Build history of the part. All positions in model axes, mm. Face numbers are marked on the shaded views. Coordinates: 2 decimals unless noted, no trailing zeros. Order: outer loops, then holes, each group sorted by start corner. A loop starts at its lowest first (then second) coordinate and runs counter-clockwise, first axis right, second up. Notation, with made-up numbers: (45.5, -31) -> (73.5, -31) arc R29 cw to (73.5, -8) -> close; hole circle Ø10 at (66, 49). An arc over 180 degrees is marked (long way). Write each question's results on one line, items separated by ' | '.
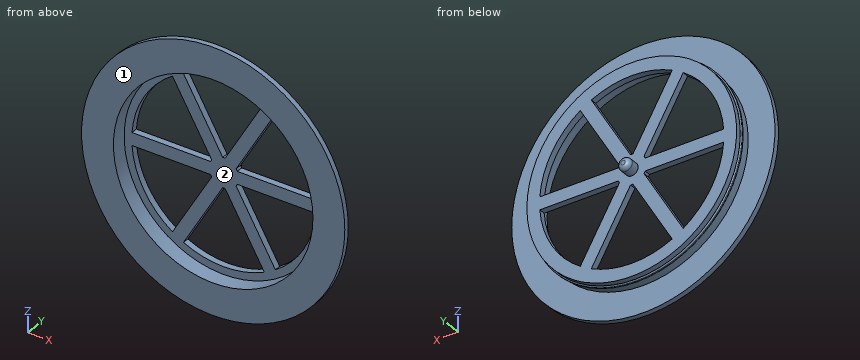
from build123d import *

# Parameters (mm, degrees)
SKETCH1_R           = 31
SKETCH1_R_2         = 23.5
BOSS_EXTRUDE1_DEPTH = 1.2
SKETCH2_R           = 24.7
SKETCH2_R_2         = 23.5
BOSS_EXTRUDE2_DEPTH = 4
BOSS_EXTRUDE3_START = -2
SKETCH3_R           = 25
SKETCH3_R_2         = 24.7
BOSS_EXTRUDE3_DEPTH = 0.75
FILLET1_R           = 0.25
BOSS_EXTRUDE4_DEPTH = 1.5
SKETCH5_R           = 24.7
SKETCH5_R_2         = 21.7
BOSS_EXTRUDE5_DEPTH = 1.5
SKETCH6_R           = 1.5
BOSS_EXTRUDE6_DEPTH = 3
FILLET2_R           = 1


with BuildPart() as part:
    # Sketch1 → Boss-Extrude1 (new body)
    with BuildSketch(Plane(origin=(0, 0, 0), x_dir=(1, 0, 0), z_dir=(0, 1, 0))):
        Circle(SKETCH1_R)
        Circle(SKETCH1_R_2, mode=Mode.SUBTRACT)
    extrude(amount=BOSS_EXTRUDE1_DEPTH)

    # Sketch2 → Boss-Extrude2 (add)
    with BuildSketch(Plane(origin=(0, 1.2, 0), x_dir=(1, 0, 0), z_dir=(0, 1, 0))):
        Circle(SKETCH2_R)
        Circle(SKETCH2_R_2, mode=Mode.SUBTRACT)
    extrude(amount=BOSS_EXTRUDE2_DEPTH)

    # Sketch3 → Boss-Extrude3 (add)
    with BuildSketch(Plane(origin=(0, 5.2, 0), x_dir=(1, 0, 0), z_dir=(0, 1, 0)).offset(BOSS_EXTRUDE3_START)):
        Circle(SKETCH3_R)
        Circle(SKETCH3_R_2, mode=Mode.SUBTRACT)
    extrude(amount=BOSS_EXTRUDE3_DEPTH)

    # Fillet1
    fillet1_edges = [part.edges().sort_by_distance(p)[0] for p in [
        (-25, 3.95, 0),
        (-25, 3.2, 0),
    ]]
    fillet(fillet1_edges, radius=FILLET1_R)

    # Sketch4 → Boss-Extrude4 (add)
    with BuildSketch(Plane(origin=(0, 5.2, 0), x_dir=(1, 0, 0), z_dir=(0, 1, 0))):
        with BuildLine():
            ThreePointArc((11.028167579, -22.101346562), (12.35, -21.390827473), (13.626243791, -20.601346562))
            Line((13.626243791, -20.601346562), (2.880176936, -1.988612788))
            ThreePointArc((2.880176936, -1.988612788), (3.031088913, -1.75), (3.16227766, -1.5))
            Line((3.16227766, -1.5), (24.65441137, -1.5))
            ThreePointArc((24.65441137, -1.5), (24.7, 0), (24.65441137, 1.5))
            Line((24.65441137, 1.5), (3.16227766, 1.5))
            ThreePointArc((3.16227766, 1.5), (3.030897524, 1.750331453), (2.879741939, 1.989242662))
            Line((2.879741939, 1.989242662), (13.625665835, 20.601728824))
            ThreePointArc((13.625665835, 20.601728824), (12.349399896, 21.391173932), (11.027547542, 22.101655938))
            Line((11.027547542, 22.101655938), (0.281337646, 3.488674409))
            ThreePointArc((0.281337646, 3.488674409), (-0.000382781, 3.499999979), (-0.282100724, 3.488612788))
            Line((-0.282100724, 3.488612788), (-11.028167579, 22.101346562))
            ThreePointArc((-11.028167579, 22.101346562), (-12.35, 21.390827473), (-13.626243791, 20.601346562))
            Line((-13.626243791, 20.601346562), (-2.880176936, 1.988612788))
            ThreePointArc((-2.880176936, 1.988612788), (-3.031088913, 1.75), (-3.16227766, 1.5))
            Line((-3.16227766, 1.5), (-24.65441137, 1.5))
            ThreePointArc((-24.65441137, 1.5), (-24.7, 0), (-24.65441137, -1.5))
            Line((-24.65441137, -1.5), (-3.16227766, -1.5))
            ThreePointArc((-3.16227766, -1.5), (-3.031280286, -1.749668491), (-2.88061184, -1.987982753))
            Line((-2.88061184, -1.987982753), (-13.626821737, -20.600964282))
            ThreePointArc((-13.626821737, -20.600964282), (-12.350600094, -21.390480998), (-11.028787606, -22.101037169))
            Line((-11.028787606, -22.101037169), (-0.28286371, -3.488551006))
            ThreePointArc((-0.28286371, -3.488551006), (-0.000382741, -3.499999979), (0.282100724, -3.488612788))
            Line((0.282100724, -3.488612788), (11.028167579, -22.101346562))
        make_face()
    extrude(amount=-BOSS_EXTRUDE4_DEPTH)

    # Sketch5 → Boss-Extrude5 (add)
    with BuildSketch(Plane(origin=(0, 5.2, 0), x_dir=(1, 0, 0), z_dir=(0, 1, 0))):
        Circle(SKETCH5_R)
        Circle(SKETCH5_R_2, mode=Mode.SUBTRACT)
    extrude(amount=-BOSS_EXTRUDE5_DEPTH)

    # Sketch6 → Boss-Extrude6 (add)
    with BuildSketch(Plane(origin=(0, 5.2, 0), x_dir=(1, 0, 0), z_dir=(0, 1, 0))):
        Circle(SKETCH6_R)
    extrude(amount=BOSS_EXTRUDE6_DEPTH)

    # Fillet2
    fillet2_edges = [part.edges().sort_by_distance(p)[0] for p in [
        (-1.5, 8.2, 0),
    ]]
    fillet(fillet2_edges, radius=FILLET2_R)


solid = part.part
Item 1: Drill centre lines: line 1 (Z direction, x = 0, y = 2.5); line 2 (X direction, y = 1, z = 0); line 3 (X direction, y = 4, z = -8.5). Where is each one in solid material? Low to high. Write a range as from..to.
Answer:
line 1: z = -24.7..-23.5, 23.5..24.7 | line 2: x = -31..-23.5, 23.5..31 | line 3: x = -23.19..-19.97, -6.64..-3.18, 3.17..6.64, 19.97..23.19
Item 2: Slice it at D-D, the plane z = 27.5. List the corners of the cut face in (x, y).
Answer:
outline: (-14.31, 0) -> (14.31, 0) -> (14.31, 1.2) -> (-14.31, 1.2) -> close
Item 3: Pull direction Z, two halves, no side cores. Call the marked faces 1 and 2: released by +Z, released by -Z, zero draft, split by the parting line, or undercut.
Answer:
face 1: zero draft | face 2: undercut
Item 4: Slice it at A-A, the plane x = -17.5. State how many separate pieces and enclosed holes the cut face has, and give its area (3 significant figures).
Answer:
separate pieces: 3 | enclosed holes: 0 | area: 51.4 mm^2
Item 5: Pin check, flat tips, straight feed: pin 1 (1.5 mm diameter, centred on x = 15, y = 2.5, fed in from -Z); pin 2 (0.8 mm diameter, centred on x = -9, y = 4, fed in from -Z); pin 3 (10 mm diameter, centred on x = 2.5, z = -14, fed in from -Y); pin 4 (24.5 mm diameter, centred on x = -6.5, z = -6, fed in from +Y). Stop position of each tip, or through.
Answer:
pin 1: stops at z = -20.17 | pin 2: stops at z = -23.44 | pin 3: stops at y = 3.7 | pin 4: stops at y = 8.2
